```python
from build123d import *

# Parameters (mm, degrees)
F0_R     = 20
F0_W     = 15.831889
F0_H     = 31.663778
F0_R_2   = 3.101009
F1_DEPTH = 2
F2_DEPTH = 40
F4_DEPTH = 25


with BuildPart() as f1:
    # F0 (on Top) → F1 (new body)
    with BuildSketch(Plane.XY):
        Circle(F0_R)
        with Locations((-0.272963, -0.409445)):
            Rectangle(F0_W, F0_H, mode=Mode.SUBTRACT)
        with Locations((-14.53372, 0)):
            Circle(F0_R_2, mode=Mode.SUBTRACT)
    extrude(amount=F1_DEPTH)

    # F0 (on Top) → F2 (join)
    with BuildSketch(Plane.XY):
        with Locations((-0.272963, -0.409445)):
            Rectangle(F0_W, F0_H)
    extrude(amount=F2_DEPTH)

    # F3 (on face) → F4 (cut)
    with BuildSketch(Plane(origin=(-8.188908, 0, 0), x_dir=(0, -1, 0), z_dir=(-1, 0, 0))):
        Polygon((0, 40), (16.241334, 27.432844), (16.241334, 40), align=None)
        Polygon((-15.422444, 26.886918), (0, 40), (-15.422444, 40), align=None)
    extrude(amount=-F4_DEPTH, mode=Mode.SUBTRACT)


solid = f1.part
```
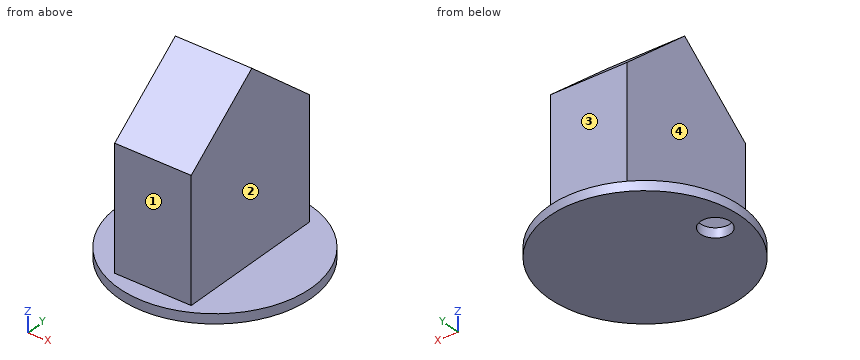
Verification items for the finished model (mm, model axes). Face numbers are marked on the shaded views. A direction names the side the tool comes from. Round coordinates to 2 decimals unless told otherwise and drop trailing zeros. Order: outer loops, then holes, each group sorted by start corner. A loop starts at its lowest first (then second) coordinate and runs counter-clockwise, first axis right, second up.
1) Cross-section at A-A, the plane x = 0. Record the cut outline in (y, z).
Geometry says:
outline: (-20, 0) - (20, 0) - (20, 2) - (15.42, 2) - (15.42, 26.89) - (0, 40) - (-16.24, 27.43) - (-16.24, 2) - (-20, 2) - close
2) Cross-section at B-B, the plane y = -6. Record the cut outline in (x, z).
Geometry says:
outline: (-19.08, 0) - (19.08, 0) - (19.08, 2) - (7.64, 2) - (7.64, 35.36) - (-8.19, 35.36) - (-8.19, 2) - (-19.08, 2) - close
3) Depth check by flat-ended pin: pin 1 (4 mm diameter, centred on x = -7, z = 19, fed in from -Y); pin 2 (16 mm diameter, centred on y = 6.5, z = 20, fed in from -X); pin 3 (2 mm diameter, centred on x = -1.5, y = -12, fed in from +Z). Enter the tip coordinate at first touch or a pass-through.
Geometry says:
pin 1: stops at y = -16.24
pin 2: stops at x = -8.19
pin 3: stops at z = 31.49
4) Material ranges on line 1 (X direction, y = 4.5, z = 16.5); line 2 (Z direction, x = 12, y = -2); line 3 (Y direction, x = -4.5, z = 7), recorded low to high.
Geometry says:
line 1: x = -8.19 to 7.64
line 2: z = 0 to 2
line 3: y = -16.24 to 15.42
5) Cross-section at D-D, the plane x = -14.5. Record the cut outline in (y, z), plus the area to 3 significant figures.
Geometry says:
outline: (-13.77, 0) - (-3.1, 0) - (-3.1, 2) - (-13.77, 2) - close; (3.1, 0) - (13.77, 0) - (13.77, 2) - (3.1, 2) - close
area: 42.7 mm2
6) Cross-section at C-C, the plane z = 4.5. Record the cut outline in (x, y).
Geometry says:
outline: (-8.19, -16.24) - (7.64, -16.24) - (7.64, 15.42) - (-8.19, 15.42) - close
7) Tool access check on the marked faces 1, 2, 3 and 4. Record the directions out of +Z, -Z, +X, -X, +Y, -Y that give a thin tool (end or side, any length) a straight path to the whole face; none if there is none.
Geometry says:
face 1: +Z, +X, -X, -Y
face 2: +Z, +X, +Y, -Y
face 3: +Z, +X, -X, +Y
face 4: +Z, -X, +Y, -Y
